Study the drawing (mm; zero at the part's minimum x, y, z) and answer. Give positions to 0.01 mm unless a question says otherwise; leave off trailing zeros. Loops run counter-clockwise (first coordinate to the right, second up) from the corner with the lowest first, then second, coordinate; pieces in that order, holes last. Notation, with made-up numbers: M 51.25,61 L 110.25,61 A34 ccw 110.25,100 Z; hole C 16.25,41 d5. An arc over 180 degrees is marked long. Return JSON: item names as keys, results as strings.
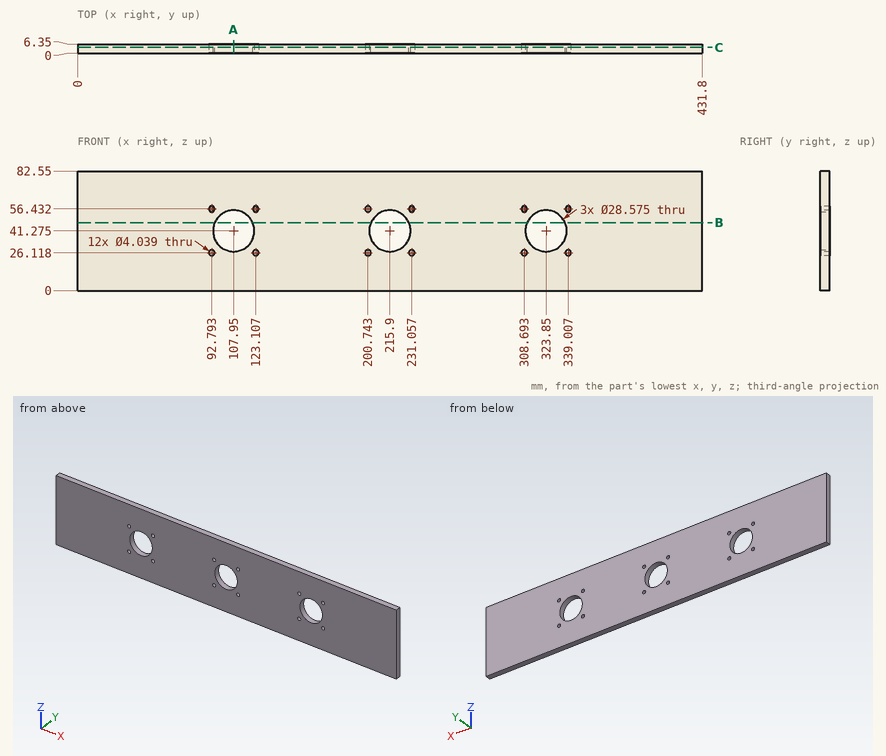
(1) The part is cut by section A-A (x = 107.95). Determine the outline of the cut face in (y, z), and give its area (3 significant figures).
Values follow:
{"outline": "M 0,0 L 6.35,0 L 6.35,26.99 L 0,26.99 Z; M 0,55.56 L 6.35,55.56 L 6.35,82.55 L 0,82.55 Z", "area": "343 mm²"}
(2) The part is cut by section B-B (z = 47). Determine the outline of the cut face in (x, y).
Values follow:
{"outline": "M 0,0 L 94.86,0 L 94.86,6.35 L 0,6.35 Z; M 121.04,0 L 202.81,0 L 202.81,6.35 L 121.04,6.35 Z; M 228.99,0 L 310.76,0 L 310.76,6.35 L 228.99,6.35 Z; M 336.94,0 L 431.8,0 L 431.8,6.35 L 336.94,6.35 Z"}
(3) The part is cut by section C-C (y = 4). Give the number of separate pieces and of enclosed holes in the cut face, and give its area (3 significant figures).
Values follow:
{"separate pieces": "1", "enclosed holes": "15", "area": "33,600 mm²"}
(4) Straight lines are drawn through the part: line 1 along X through (y, z) = (3.75, 42.5) (1 decimal); line 2 along X through (y, z) = (5.25, 35.5). For each, find the intervals that lie inside material, in ascending order.
Values follow:
{"line 1": "0 to 93.7, 122.2 to 201.7, 230.1 to 309.6, 338.1 to 431.8", "line 2": "0 to 94.88, 121.02 to 202.83, 228.97 to 310.78, 336.92 to 431.8"}
